from build123d import *

# Parameters (mm, degrees)
SKETCH1_R           = 14
BOSS_EXTRUDE1_DEPTH = 4
SKETCH2_R           = 12.5
CUT_EXTRUDE1_DEPTH  = 3
CHAMFER2_SIZE       = 2
CUT_EXTRUDE2_START  = -3
CUT_EXTRUDE2_DEPTH  = 3
FILLET2_R           = 1
SKETCH4_R           = 2.5
CUT_EXTRUDE3_DEPTH  = 3


with BuildPart() as part:
    # Sketch1 → Boss-Extrude1 (new body)
    with BuildSketch(Plane(origin=(0, 0, 0), x_dir=(1, 0, 0), z_dir=(0, 1, 0))):
        with Locations(Location((0, 0, 0), (0, 0, 270))):
            Circle(SKETCH1_R)
    extrude(amount=BOSS_EXTRUDE1_DEPTH)

    # Sketch2 → Cut-Extrude1 (cut)
    with BuildSketch(Plane.XZ):
        with Locations(Location((0, 0, 0), (0, 0, 270))):
            Circle(SKETCH2_R)
    extrude(amount=-CUT_EXTRUDE1_DEPTH, mode=Mode.SUBTRACT)

    # Chamfer2
    chamfer2_edges = [part.edges().sort_by_distance(p)[0] for p in [
        (0, 4, -14),
        (0, 3, 12.5),
    ]]
    chamfer(chamfer2_edges, length=CHAMFER2_SIZE)

    # Sketch3 → Cut-Extrude2 (cut)
    with BuildSketch(Plane(origin=(0, 4, 0), x_dir=(1, 0, 0), z_dir=(0, 1, 0)).offset(CUT_EXTRUDE2_START)):
        with BuildLine():
            Line((-11.736694594, 2.5), (-13.774977314, 2.5))
            ThreePointArc((-13.774977314, 2.5), (-14, 0), (-13.774977314, -2.5))
            Line((-13.774977314, -2.5), (-11.736694594, -2.5))
            ThreePointArc((-11.736694594, -2.5), (-12, 0), (-11.736694594, 2.5))
        make_face()
        with BuildLine():
            Line((-8.5, 2.5), (-11.736694594, 2.5))
            ThreePointArc((-11.736694594, 2.5), (-12, 0), (-11.736694594, -2.5))
            Line((-11.736694594, -2.5), (-8.5, -2.5))
            Line((-8.5, -2.5), (-8.5, 2.5))
        make_face()
        with BuildLine():
            ThreePointArc((-6.531329383, 10.066863289), (-8.485281374, 8.485281374), (-10.066863289, 6.531329383))
            Line((-10.066863289, 6.531329383), (-7.778174593, 4.242640687))
            Line((-7.778174593, 4.242640687), (-4.242640687, 7.778174593))
            Line((-4.242640687, 7.778174593), (-6.531329383, 10.066863289))
        make_face()
        with BuildLine():
            Line((-11.508146822, 7.972612916), (-10.066863289, 6.531329383))
            ThreePointArc((-10.066863289, 6.531329383), (-8.485281374, 8.485281374), (-6.531329383, 10.066863289))
            Line((-6.531329383, 10.066863289), (-7.972612916, 11.508146822))
            ThreePointArc((-7.972612916, 11.508146822), (-9.899494937, 9.899494937), (-11.508146822, 7.972612916))
        make_face()
        with BuildLine():
            ThreePointArc((2.5, 11.736694594), (0, 12), (-2.5, 11.736694594))
            Line((-2.5, 11.736694594), (-2.5, 8.5))
            Line((-2.5, 8.5), (2.5, 8.5))
            Line((2.5, 8.5), (2.5, 11.736694594))
        make_face()
        with BuildLine():
            Line((-2.5, 13.774977314), (-2.5, 11.736694594))
            ThreePointArc((-2.5, 11.736694594), (0, 12), (2.5, 11.736694594))
            Line((2.5, 11.736694594), (2.5, 13.774977314))
            ThreePointArc((2.5, 13.774977314), (0, 14), (-2.5, 13.774977314))
        make_face()
        with BuildLine():
            ThreePointArc((10.066863289, 6.531329383), (8.485281374, 8.485281374), (6.531329383, 10.066863289))
            Line((6.531329383, 10.066863289), (4.242640687, 7.778174593))
            Line((4.242640687, 7.778174593), (7.778174593, 4.242640687))
            Line((7.778174593, 4.242640687), (10.066863289, 6.531329383))
        make_face()
        with BuildLine():
            Line((7.972612916, 11.508146822), (6.531329383, 10.066863289))
            ThreePointArc((6.531329383, 10.066863289), (8.485281374, 8.485281374), (10.066863289, 6.531329383))
            Line((10.066863289, 6.531329383), (11.508146822, 7.972612916))
            ThreePointArc((11.508146822, 7.972612916), (9.899494937, 9.899494937), (7.972612916, 11.508146822))
        make_face()
        with BuildLine():
            ThreePointArc((12, 0), (11.933992105, 1.256913853), (11.736694594, 2.5))
            Line((11.736694594, 2.5), (8.5, 2.5))
            Line((8.5, 2.5), (8.5, -2.5))
            Line((8.5, -2.5), (11.736694594, -2.5))
            ThreePointArc((11.736694594, -2.5), (11.933992105, -1.256913853), (12, 0))
        make_face()
        with BuildLine():
            Line((13.774977314, 2.5), (11.736694594, 2.5))
            ThreePointArc((11.736694594, 2.5), (11.933992105, 1.256913853), (12, 0))
            ThreePointArc((12, 0), (11.933992105, -1.256913853), (11.736694594, -2.5))
            Line((11.736694594, -2.5), (13.774977314, -2.5))
            ThreePointArc((13.774977314, -2.5), (14, 0), (13.774977314, 2.5))
        make_face()
        with BuildLine():
            Line((4.242640687, -7.778174593), (6.531329383, -10.066863289))
            ThreePointArc((6.531329383, -10.066863289), (8.485281374, -8.485281374), (10.066863289, -6.531329383))
            Line((10.066863289, -6.531329383), (7.778174593, -4.242640687))
            Line((7.778174593, -4.242640687), (4.242640687, -7.778174593))
        make_face()
        with BuildLine():
            ThreePointArc((10.066863289, -6.531329383), (8.485281374, -8.485281374), (6.531329383, -10.066863289))
            Line((6.531329383, -10.066863289), (7.972612916, -11.508146822))
            ThreePointArc((7.972612916, -11.508146822), (9.899494937, -9.899494937), (11.508146822, -7.972612916))
            Line((11.508146822, -7.972612916), (10.066863289, -6.531329383))
        make_face()
        with BuildLine():
            Line((-2.5, -8.5), (-2.5, -11.736694594))
            ThreePointArc((-2.5, -11.736694594), (0, -12), (2.5, -11.736694594))
            Line((2.5, -11.736694594), (2.5, -8.5))
            Line((2.5, -8.5), (-2.5, -8.5))
        make_face()
        with BuildLine():
            ThreePointArc((2.5, -11.736694594), (0, -12), (-2.5, -11.736694594))
            Line((-2.5, -11.736694594), (-2.5, -13.774977314))
            ThreePointArc((-2.5, -13.774977314), (0, -14), (2.5, -13.774977314))
            Line((2.5, -13.774977314), (2.5, -11.736694594))
        make_face()
        with BuildLine():
            Line((-7.778174593, -4.242640687), (-10.066863289, -6.531329383))
            ThreePointArc((-10.066863289, -6.531329383), (-8.485281374, -8.485281374), (-6.531329383, -10.066863289))
            Line((-6.531329383, -10.066863289), (-4.242640687, -7.778174593))
            Line((-4.242640687, -7.778174593), (-7.778174593, -4.242640687))
        make_face()
        with BuildLine():
            ThreePointArc((-6.531329383, -10.066863289), (-8.485281374, -8.485281374), (-10.066863289, -6.531329383))
            Line((-10.066863289, -6.531329383), (-11.508146822, -7.972612916))
            ThreePointArc((-11.508146822, -7.972612916), (-9.899494937, -9.899494937), (-7.972612916, -11.508146822))
            Line((-7.972612916, -11.508146822), (-6.531329383, -10.066863289))
        make_face()
    extrude(amount=CUT_EXTRUDE2_DEPTH, mode=Mode.SUBTRACT)

    # Fillet2
    fillet2_edges = [part.edges().sort_by_distance(p)[0] for p in [
        (4.242640687, 3.5, -7.778174593),
        (7.778174593, 3.5, -4.242640687),
        (8.5, 3.5, -2.5),
        (8.5, 3.5, 2.5),
        (7.778174593, 3.5, 4.242640687),
        (4.242640687, 3.5, 7.778174593),
        (2.5, 3.5, 8.5),
        (-2.5, 3.5, 8.5),
        (-4.242640687, 3.5, 7.778174593),
        (-7.778174593, 3.5, 4.242640687),
        (-8.5, 3.5, -2.5),
        (-8.5, 3.5, 2.5),
        (-4.242640687, 3.5, -7.778174593),
        (-7.778174593, 3.5, -4.242640687),
        (2.5, 3.5, -8.5),
        (-2.5, 3.5, -8.5),
    ]]
    fillet(fillet2_edges, radius=FILLET2_R)

    # Sketch4 → Cut-Extrude3 (cut)
    with BuildSketch(Plane(origin=(0, 4, 0), x_dir=(1, 0, 0), z_dir=(0, 1, 0))):
        with Locations(Location((0, 0, 0), (0, 0, 270))):
            Circle(SKETCH4_R)
    extrude(amount=-CUT_EXTRUDE3_DEPTH, mode=Mode.SUBTRACT)


solid = part.part
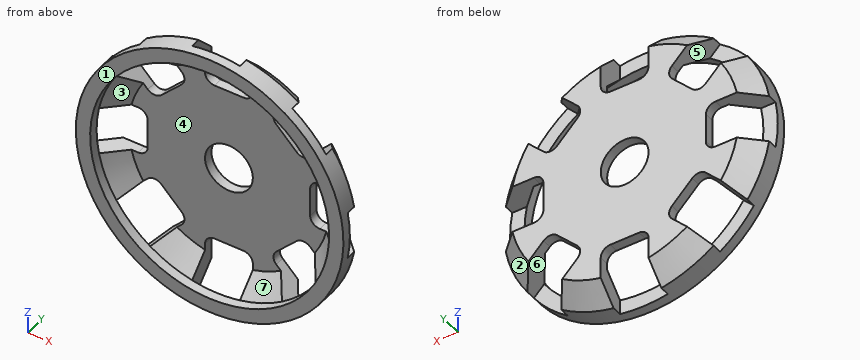
CAD build for the part. Positions are in the model's coordinates, mm. Face numbers are marked on the shaded views. A direction names the side the tool comes from. Round coordinates to 2 decimals unless told otherwise and drop trailing zeros. Write each loop counter-clockwise with the first axis right and the second up, starting at its lowest first coordinate (ties: lowest second). Pieces come first, ordered by that corner, then holes. Notation, with made-up numbers: M 75.5,-10.5 L 95.5,-10.5 A28 ccw 95.5,28.5 Z; hole C 29,38.5 d11. An arc over 180 degrees is marked long. Put each result on its own line as item: value. Start each with the question number.
1) Pull direction X, two halves, no side cores. Call the marked faces 1, 2, 3 and 4: pulls with the +X half, pulls with the -X half, needs draft (parallel to the pull), parting line crosses it, or undercut.
2) Saw through at D-D, the plane y = 0.55. Write the cut outline in (x, z), and give its area (3 significant figures).
3) Saw through at B-B, the plane z = 0. Write the cut outline in (x, y), and give its area (3 significant figures).
4) Pin check, flat tips, straight feed: pin 1 Ø0.9 at (x, y) = (-12, 2) entering from +Z; pin 2 Ø1 at (y, z) = (1, -6.5) entering from -X; pin 3 Ø2 at (y, z) = (0.5, 6.5) entering from +X; pin 4 Ø4 at (x, z) = (0, 0) entering from -Y. Stop position of each tip, or through.
5) Saw through at A-A, the plane x = 0. Write the cut outline in (y, z).
6) 3-axis set-ups, long thin cutter, end or side, ignore diameter. For the marked faces 5, 6 and 7: which of +Z, -Z, +X, -X, +Y, -Y reach the whole face in a straight line?
7) Drill centre lines: probe 1 along X at (y, z) = (3.5, 0); probe 2 along X at (y, z) = (0.2, 0); probe 3 along Z at (x, y) = (-6, 3.4). Where is each one in solid material? Low to high. Write a range as [from, to].
8) Saw through at C-C, the plane y = 2.55. Count the separate pieces of the cut face and the enclosed holes in it, and give its area (3 significant figures).
Resolved:
1. face 1: needs draft
1. face 2: pulls with the +X half
1. face 3: undercut
1. face 4: undercut
2. outline: C 0,0 d28; hole C 0,0 d25
2. area: 125 mm²
3. outline: M -14,0 L -12.5,0 L -12.5,1 L -14,1 Z; M -8.5,3 L -2.5,3 L -2.5,4 L -8.5,4 Z; M 2.5,3 L 8.5,3 L 8.5,4 L 2.5,4 Z; M 12.5,0 L 14,0 L 14,1 L 12.5,1 Z
3. area: 15.0 mm²
4. pin 1: z = 7.91
4. pin 2: x = -12.65
4. pin 3: x = 12.87
4. pin 4: through
5. outline: M 0,-14 L 1,-14 L 1,-12.5 L 0,-12.5 Z; M 0,12.5 L 1,12.5 L 1,14 L 0,14 Z; M 3,-8.5 L 4,-8.5 L 4,-2.5 L 3,-2.5 Z; M 3,2.5 L 4,2.5 L 4,8.5 L 3,8.5 Z
6. face 5: -X, +Y
6. face 6: -Z, +Y
6. face 7: -Y
7. probe 1: [-8.5, -2.5], [2.5, 8.5]
7. probe 2: [-14, -12.5], [12.5, 14]
7. probe 3: [-11.08, -9.54], [-6.02, 6.02], [9.54, 11.08]
8. separate pieces: 8
8. enclosed holes: 0
8. area: 90.9 mm²
